```python
from build123d import *

# Parameters (mm, degrees)
F0_W     = 68.58
F0_H     = 83.82
F1_DEPTH = 35.56
F2_R     = 0.508
F3_T     = -1.27
F4_R     = 0.508


with BuildPart() as f1:
    # F0 (on Top) → F1 (new body)
    with BuildSketch(Plane.XY):
        with Locations((36.83, 44.45)):
            Rectangle(F0_W, F0_H)
    extrude(amount=F1_DEPTH)

    # F2
    f2_edges = [f1.edges().sort_by_distance(p)[0] for p in [
        (71.12, 2.54, 17.78),
        (71.12, 86.36, 17.78),
        (2.54, 2.54, 17.78),
        (2.54, 86.36, 17.78),
        (71.12, 44.45, 0),
        (2.54, 44.45, 0),
        (36.83, 2.54, 0),
        (36.83, 86.36, 0),
    ]]
    fillet(f2_edges, radius=F2_R)

    # F3
    f3_openings = [f1.faces().sort_by_distance(p)[0] for p in [
        (36.83, 44.45, 35.56),
    ]]
    offset(amount=F3_T, openings=f3_openings)

    # F4
    f4_edges = [f1.edges().sort_by_distance(p)[0] for p in [
        (3.81, 3.81, 18.415),
        (3.81, 85.09, 18.415),
        (69.85, 85.09, 18.415),
        (69.85, 3.81, 18.415),
    ]]
    fillet(f4_edges, radius=F4_R)


solid = f1.part
```
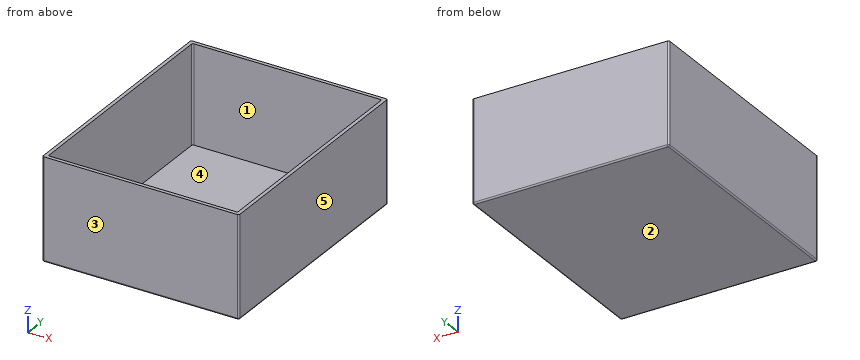
Geometry check sheet. Reference: the model listing, model coordinates, mm. Face numbers are marked on the shaded views. A direction names the side the tool comes from. Give positions to 0.01 mm unless a question says otherwise; leave off trailing zeros. Loops run counter-clockwise (first coordinate to the right, second up) from the corner with the lowest first, then second, coordinate; pieces in that order, holes last. Notation, with made-up numbers: M 52.25,18 L 59.25,18 A20 ccw 59.25,25 Z; hole C 45.5,70.25 d11. An arc over 180 degrees is marked long. Write item = value, one per line.
(1) Gauge pin test, flat end, axial feed: pin 1 Ø12 at (x, y) = (33.5, 72.5) entering from +Z. Record the tip position at first contact, or that the pin passes through.
Answer below:
pin_1 = 1.27
(2) Sectioned sample at A-A, the plane z = 21. Record the cut outline in (x, y).
Answer below:
outline = M 2.54,3.05 A0.51 ccw 3.05,2.54 L 70.61,2.54 A0.51 ccw 71.12,3.05 L 71.12,85.85 A0.51 ccw 70.61,86.36 L 3.05,86.36 A0.51 ccw 2.54,85.85 Z; hole M 3.81,4.32 A0.51 ccw 4.32,3.81 L 69.34,3.81 A0.51 ccw 69.85,4.32 L 69.85,84.58 A0.51 ccw 69.34,85.09 L 4.32,85.09 A0.51 ccw 3.81,84.58 Z
(3) Release check for a two-part mould opening along X. For the marked faces 3, 4 and 5 record: released by +X, released by -X, zero draft, split by the parting line, or undercut.
Answer below:
face_3 = zero draft
face_4 = undercut
face_5 = released by +X
(4) Sectioned sample at B-B, the plane x = 8.5. Record the cut outline in (y, z).
Answer below:
outline = M 2.54,0.51 A0.51 ccw 3.05,0 L 85.85,0 A0.51 ccw 86.36,0.51 L 86.36,35.56 L 85.09,35.56 L 85.09,1.27 L 3.81,1.27 L 3.81,35.56 L 2.54,35.56 Z
(5) Tool access check on the marked faces 1 and 2. Record the directions out of +Z, -Z, +X, -X, +Y, -Y that give a thin tool (end or side, any length) a straight path to the whole face; none if there is none.
Answer below:
face_1 = +Z
face_2 = -Z, +X, -X, +Y, -Y
(6) Sectioned sample at C-C, the plane y = 15.5. Record the cut outline in (x, z), plus the area to 3 significant figures.
Answer below:
outline = M 2.54,0.51 A0.51 ccw 3.05,0 L 70.61,0 A0.51 ccw 71.12,0.51 L 71.12,35.56 L 69.85,35.56 L 69.85,1.27 L 3.81,1.27 L 3.81,35.56 L 2.54,35.56 Z
area = 174 mm2
(7) Material ranges on line 1 (Y direction, x = 34, z = 11); line 2 (X direction, y = 59, z = 12); line 3 (Z direction, x = 39.5, y = 56), recorded low to high. Write a range as [from, to].
Answer below:
line_1 = [2.54, 3.81], [85.09, 86.36]
line_2 = [2.54, 3.81], [69.85, 71.12]
line_3 = [0, 1.27]
